Verification items for this drawing (mm, ordinates from the low corner). Round coordinates to 2 decimals unless told otherwise and drop trailing zeros. Loops run counter-clockwise (first coordinate to the right, second up) from the corner with the lowest first, then second, coordinate; pieces in that order, holes last. Notation, with made-up numbers: M -5.75,-3 L 28.25,-3 A17 cw 28.25,8 Z; hole C -27,-23.75 d1. An arc over 180 degrees is marked long. Use one line per item in the form item = value. Start each with the question number.
1. Cross-section at B-B (y = 15). Record the boundary of the cut face in (x, z).
2. Material ranges on line 1 (X direction, y = 16, z = 3.25); line 2 (Y direction, x = 199.5, z = 3.4); line 3 (X direction, y = 56.5, z = 2.6), recorded low to high.
3. Cross-section at C-C (x = 15.5). Record the boundary of the cut face in (y, z).
4. Cross-section at A-A (z = 1.5). Record the boundary of the cut face in (x, y).
5. Go/stop test with flat-tipped pins: pin 1 (3 mm diameter, centred on x = 200, z = 5, fed in from +Y); pin 2 (1.8 mm diameter, centred on x = 224, z = 2, fed in from -Y); pin 3 (3 mm diameter, centred on x = 3.5, z = 4, fed in from +Y); pin 4 (1.8 mm diameter, centred on y = 17, z = 2.5, fed in from -X). Record where each tip stops, or that it passes through.
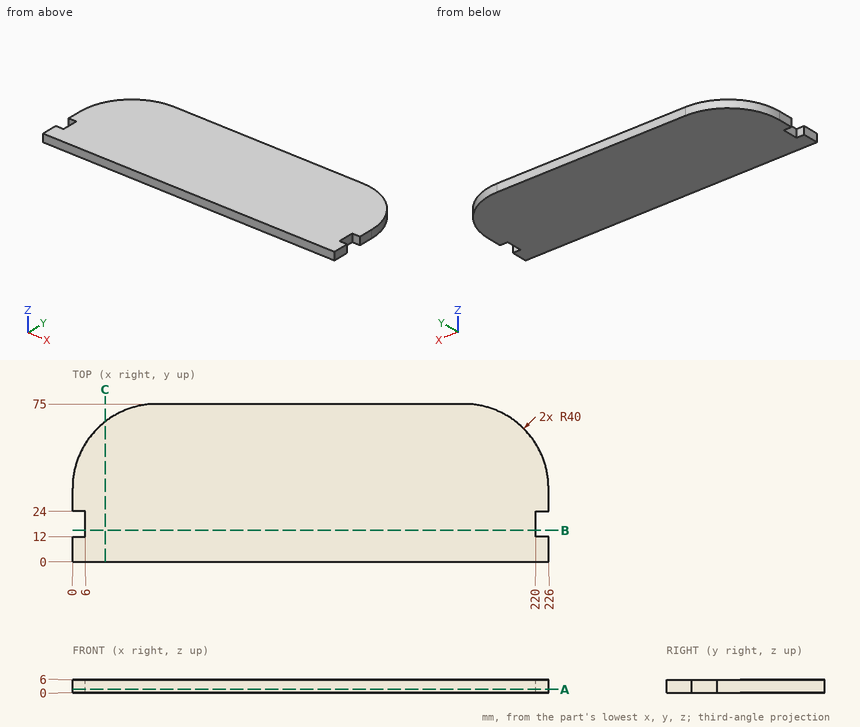
Reported:
q1.outline = M 6,0 L 220,0 L 220,6 L 6,6 Z
q2.line_1 = 6 to 220
q2.line_2 = 0 to 72.65
q2.line_3 = 6.27 to 219.73
q3.outline = M 0,0 L 66.62,0 L 66.62,6 L 0,6 Z
q4.outline = M 0,0 L 226,0 L 226,12 L 220,12 L 220,24 L 226,24 L 226,35 A40 ccw 186,75 L 40,75 A40 ccw 0,35 L 0,24 L 6,24 L 6,12 L 0,12 Z
q5.pin_1 = 73
q5.pin_2 = 0
q5.pin_3 = 54.36
q5.pin_4 = 6
